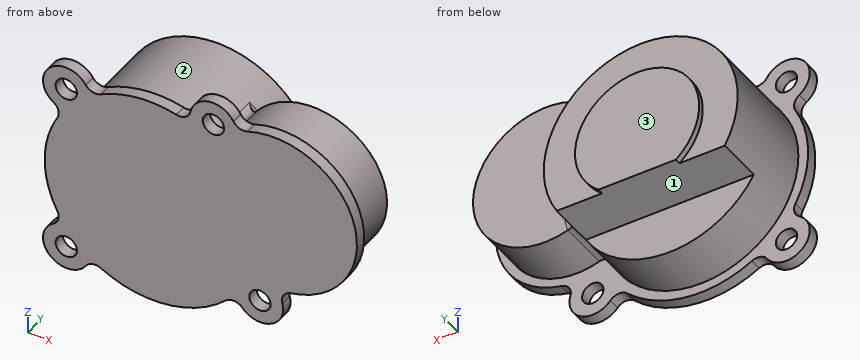
from build123d import *

# Parameters (mm, degrees)
BOSS_EXTRUDE1_DEPTH = 6
SKETCH2_R           = 5.5
CUT_EXTRUDE1_DEPTH  = 6
SKETCH3_R           = 50
BOSS_EXTRUDE2_DEPTH = 50
SKETCH4_R           = 37.5
BOSS_EXTRUDE3_DEPTH = 26
SKETCH5_R           = 32
BOSS_EXTRUDE4_DEPTH = 3
FILLET2_R           = 6
FILLET3_R           = 6
FILLET4_R           = 5
CUT_EXTRUDE2_START  = -27
CUT_EXTRUDE2_DEPTH  = 27


with BuildPart() as part:
    # Sketch1 → Boss-Extrude1 (new body)
    with BuildSketch(Plane(origin=(0, 0, 0), x_dir=(1, 0, 0), z_dir=(0, 1, 0))):
        with BuildLine():
            ThreePointArc((21.211789327, -50.745048956), (28.860136885, -67.581936782), (43.965179902, -56.913493246))
            ThreePointArc((43.965179902, -56.913493246), (104.875389558, -29.654145663), (62.597817721, 21.976587342))
            ThreePointArc((62.597817721, 21.976587342), (62.107138398, 42.329707672), (44.037643352, 32.949749135))
            ThreePointArc((44.037643352, 32.949749135), (8.49481412, 54.340023308), (-31.880473469, 44.817802394))
            ThreePointArc((-31.880473469, 44.817802394), (-52.325901808, 52.325901808), (-44.817802394, 31.880473469))
            ThreePointArc((-44.817802394, 31.880473469), (-55, 0), (-44.817802394, -31.880473469))
            ThreePointArc((-44.817802394, -31.880473469), (-52.325901808, -52.325901808), (-31.880473469, -44.817802394))
            ThreePointArc((-31.880473469, -44.817802394), (-6.102316632, -54.660421986), (21.211789327, -50.745048956))
        make_face()
    extrude(amount=BOSS_EXTRUDE1_DEPTH)

    # Sketch2 → Cut-Extrude1 (cut)
    with BuildSketch(Plane(origin=(0, 6, 0), x_dir=(1, 0, 0), z_dir=(0, 1, 0))):
        with Locations(Location((56, 32, 0), (0, 0, 270))):
            Circle(SKETCH2_R)
        with Locations(Location((-43.840620434, 43.840620434, 0), (0, 0, 270))):
            Circle(SKETCH2_R)
        with Locations(Location((-43.840620434, -43.840620434, 0), (0, 0, 270))):
            Circle(SKETCH2_R)
        with Locations(Location((32, -56, 0), (0, 0, 270))):
            Circle(SKETCH2_R)
    extrude(amount=-CUT_EXTRUDE1_DEPTH, mode=Mode.SUBTRACT)

    # Sketch3 → Boss-Extrude2 (add)
    with BuildSketch(Plane(origin=(0, 6, 0), x_dir=(1, 0, 0), z_dir=(0, 1, 0))):
        with Locations(Location((0, 0, 0), (0, 0, 270))):
            Circle(SKETCH3_R)
    extrude(amount=BOSS_EXTRUDE2_DEPTH)

    # Sketch4 → Boss-Extrude3 (add)
    with BuildSketch(Plane(origin=(0, 6, 0), x_dir=(1, 0, 0), z_dir=(0, 1, 0))):
        with Locations((64, -20)):
            Circle(SKETCH4_R)
    extrude(amount=BOSS_EXTRUDE3_DEPTH)

    # Sketch5 → Boss-Extrude4 (add)
    with BuildSketch(Plane(origin=(0, 56, 0), x_dir=(1, 0, 0), z_dir=(0, 1, 0))):
        with Locations(Location((0, 0, 0), (0, 0, 270))):
            Circle(SKETCH5_R)
    extrude(amount=BOSS_EXTRUDE4_DEPTH)

    # Fillet2
    fillet2_edges = [part.edges().sort_by_distance(p)[0] for p in [
        (44.037643352, 3, -32.949749135),
    ]]
    fillet(fillet2_edges, radius=FILLET2_R)

    # Fillet3
    fillet3_edges = [part.edges().sort_by_distance(p)[0] for p in [
        (21.211789327, 3, 50.745048956),
        (-31.880473469, 3, 44.817802394),
        (-44.817802394, 3, 31.880473469),
        (-44.817802394, 3, -31.880473469),
        (-31.880473469, 3, -44.817802394),
        (62.597817721, 3, -21.976587342),
        (43.965179902, 3, 56.913493246),
    ]]
    fillet(fillet3_edges, radius=FILLET3_R)

    # Fillet4
    fillet4_edges = [part.edges().sort_by_distance(p)[0] for p in [
        (47.723998902, 32, 14.913749657),
        (48.021654026, 19, -13.925542883),
        (31.547740992, 19, 38.790978827),
    ]]
    fillet(fillet4_edges, radius=FILLET4_R)

    # Sketch6 → Cut-Extrude2 (cut)
    with BuildSketch(Plane(origin=(0, 59, 0), x_dir=(1, 0, 0), z_dir=(0, 1, 0)).offset(CUT_EXTRUDE2_START)):
        with BuildLine():
            Line((0, 25), (43.301270189, 25))
            ThreePointArc((43.301270189, 25), (0, 50), (-43.301270189, 25))
            Line((-43.301270189, 25), (0, 25))
        make_face()
    extrude(amount=CUT_EXTRUDE2_DEPTH, mode=Mode.SUBTRACT)


solid = part.part
Read the model definition and answer for the solid it produces. Units are mm, in the model's axes. Face numbers are marked on the shaded views. A direction names the side the tool comes from. Give positions to 0.01 mm unless a question says otherwise; leave off trailing zeros. Write each loop counter-clockwise with the first axis right and the second up, starting at its lowest first coordinate (ties: lowest second). Pieces come first, ordered by that corner, then holes. Notation, with made-up numbers: (-34.5, 78) -> (1.5, 78) arc R30 ccw to (1.5, 113) -> close; hole circle Ø7 at (-10.75, 25.5). An arc over 180 degrees is marked (long way). Answer as a JSON object with one key per item and string values. Group by question number.
1) Find section C-C (z = 0). Write down the section's boundary in (x, y).
2) A tool of negligible diameter and unlimited length cuts with its end or side. For the marked faces 1, 2 and 3, from which of +Z, -Z, +X, -X, +Y, -Y can it reach the whole face along a straight path? Write none if from no direction.
3) Consider L1, parallel to Y at x = 95, z = 12; L2, parallel to Y at x = -43, z = -1.5; L3, parallel to Z at x = 30.5, y = 33. Determine where each line is inside the solid, lowest interval first. Write a range as from..to.
4) Find section B-B (y = 44). Write down the section's boundary in (x, z).
5) Each of these flat-tipped pins is pushed along its axis until it touches: P1, Ø17.5, axis at x = -43.84, z = 43.84, coming from the +Y side; P2, Ø1.5, axis at x = 17.5, y = 20.5, coming from the -Z side; P3, Ø1, axis at y = 16.5, z = 37, coming from the +X side; P4, Ø14.5, axis at x = -43.84, z = -43.84, coming from the -Y side. Where does it stop, or does it pass through?
6) Find section A-A (x = 64). Write down the section's boundary in (y, z), and give its area (3 significant figures).
Values follow:
{
 "1": {"outline": "(-55, 0) -> (100.93, 0) -> (100.93, 6) -> (95.72, 6) -> (95.72, 32) -> (55, 32) arc R5 cw to (50, 37) -> (50, 56) -> (32, 56) -> (32, 59) -> (-32, 59) -> (-32, 56) -> (-50, 56) -> (-50, 6) -> (-55, 6) -> close"},
 "2": {"face 1": "-Z, +X, -X, +Y", "face 2": "+Y", "face 3": "+Z, -Z, +X, -X, +Y"},
 "3": {"L1": "y = 0..32", "L2": "y = 0..56", "L3": "z = -25..40.9"},
 "4": {"outline": "(-43.3, -25) -> (43.3, -25) arc R50 ccw (long way) to start"},
 "5": {"P1": "stops at y = 6", "P2": "stops at z = -47.11", "P3": "stops at x = 97.67", "P4": "stops at y = 0"},
 "6": {"outline": "(0, -40.94) -> (6, -40.94) -> (6, -17.5) -> (32, -17.5) -> (32, 57.5) -> (6, 57.5) -> (6, 62) -> (0, 62) -> close", "area": "2,570 mm2"}
}
